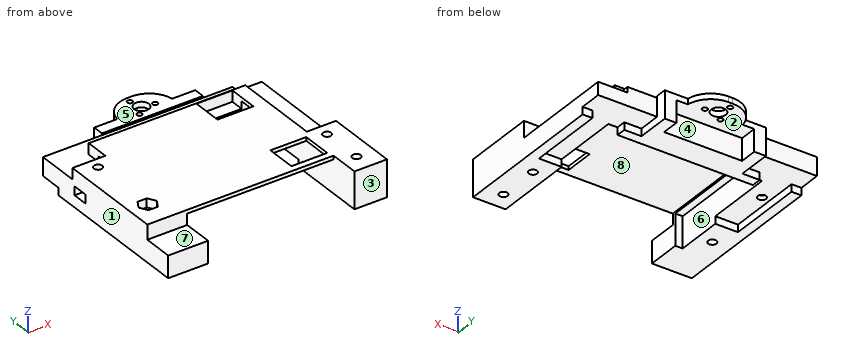
```python
from build123d import *

# Parameters (mm, degrees)
SKETCH1_R           = 6
BOSS_EXTRUDE1_DEPTH = 6
SKETCH2_W           = 27.6
SKETCH2_H           = 16.6
SKETCH2_R           = 6
SKETCH2_R_2         = 0.705
SKETCH2_R_3         = 2
BOSS_EXTRUDE2_DEPTH = 1.5
BOSS_EXTRUDE3_START = -4
BOSS_EXTRUDE3_DEPTH = 4
SKETCH5_W           = 40
SKETCH5_H           = 38.75
CUT_EXTRUDE1_DEPTH  = 50.346876803
SKETCH6_W           = 59.8
SKETCH6_H           = 40.75
BOSS_EXTRUDE4_DEPTH = 4
SKETCH7_W           = 40
SKETCH7_H           = 38.75
CUT_EXTRUDE2_DEPTH  = 3
SKETCH8_W           = 10.5
SKETCH8_H           = 8.15
CUT_EXTRUDE3_DEPTH  = 3
SKETCH8_3_W         = 9.813424901
SKETCH8_3_H         = 8.2
CUT_EXTRUDE4_DEPTH  = 1
CUT_EXTRUDE5_DEPTH  = 2
SKETCH10_W          = 8.9
SKETCH10_H          = 8.15
BOSS_EXTRUDE5_DEPTH = 4
SKETCH12_W          = 7.5
SKETCH12_H          = 1.5
CUT_EXTRUDE7_DEPTH  = 50.346876803
CUT_EXTRUDE8_DEPTH  = 2.4
CUT_EXTRUDE9_DEPTH  = 2.4
SKETCH16_R          = 1.125
CUT_EXTRUDE10_DEPTH = 50.788193884
SKETCH17_W          = 42
SKETCH17_H          = 31
CUT_EXTRUDE11_DEPTH = 8.5
SKETCH19_W          = 21.3
SKETCH19_H          = 12.25
CUT_EXTRUDE12_DEPTH = 50.141268301
SKETCH20_W          = 3.149886021
SKETCH20_H          = 7.5
SKETCH20_W_2        = 3.150113979
CUT_EXTRUDE13_DEPTH = 50.346876803
FILLET1_R           = 7
SKETCH21_W          = 5
SKETCH21_H          = 1.4
CUT_EXTRUDE14_DEPTH = 50.141268301
SKETCH22_W          = 9.813424901
SKETCH22_H          = 3.6
CUT_EXTRUDE15_DEPTH = 2
SKETCH23_W          = 3.149886021
SKETCH23_H          = 7.5
SKETCH23_W_2        = 3.150113979
CUT_EXTRUDE16_DEPTH = 50.346876803
SKETCH24_W          = 35
SKETCH24_H          = 1.4
CUT_EXTRUDE17_DEPTH = 49.713519689


# Read off the part's stored shape, not the designer's step: Boss-Extrude3
with BuildPart() as part:
    # Sketch1 → Boss-Extrude1 (new body)
    with BuildSketch(Plane.XY):
        Polygon((-10.832250172, 36.035749909), (-10.832250172, 19.435749909), (-15.532250172, 19.435749909), (-15.532250172, -1.464250091), (-24.232250172, -1.464250091), (-24.232250172, 19.435749909), (-26.932250172, 19.435749909), (-26.932250172, -23.364250091), (32.867749828, -23.364250091), (32.867749828, 19.435749909), (30.167749828, 19.435749909), (30.167749828, -1.464250091), (21.467749828, -1.464250091), (21.467749828, 19.435749909), (16.767749828, 19.435749909), (16.767749828, 36.035749909), align=None)
        with Locations((2.967749828, 29.785749909)):
            Circle(SKETCH1_R, mode=Mode.SUBTRACT)
    extrude(amount=BOSS_EXTRUDE1_DEPTH)

    # Sketch2 → Boss-Extrude2 (add)
    # profile 1 of 2: a face of its own
    with BuildSketch(Plane.XY.offset(6)):
        with Locations((2.967749828, 27.735749909)):
            Rectangle(SKETCH2_W, SKETCH2_H)
        with Locations((2.967749828, 29.785749909)):
            Circle(SKETCH2_R, mode=Mode.SUBTRACT)
    # profile 2 of 2: a face of its own
    with BuildSketch(Plane.XY.offset(6)):
        with Locations((2.967749828, 29.785749909)):
            Circle(SKETCH2_R)
        with Locations((0.732850657, 27.357741339)):
            Circle(SKETCH2_R_2, mode=Mode.SUBTRACT)
        with Locations((6.187916827, 29.064275155)):
            Circle(SKETCH2_R_2, mode=Mode.SUBTRACT)
        with Locations((1.982482071, 32.935233827)):
            Circle(SKETCH2_R_2, mode=Mode.SUBTRACT)
        with Locations((2.967749828, 29.785749909)):
            Circle(SKETCH2_R_3, mode=Mode.SUBTRACT)
    extrude(amount=BOSS_EXTRUDE2_DEPTH)

    # Boss-Extrude3 outline → Boss-Extrude3 (add)
    with BuildSketch(Plane.XY.offset(6).offset(BOSS_EXTRUDE3_START)):
        Polygon((32.867749828, 19.435749909), (32.867749828, 25.535749909), (16.767749828, 25.535749909), (16.767749828, 19.435749909), (21.467749828, 19.435749909), (21.467749828, -1.464250091), (30.167749828, -1.464250091), (30.167749828, 19.435749909), align=None)
        Polygon((-26.932250172, 25.535749909), (-26.932250172, 19.435749909), (-24.232250172, 19.435749909), (-24.232250172, -1.464250091), (-15.532250172, -1.464250091), (-15.532250172, 19.435749909), (-10.832250172, 19.435749909), (-10.832250172, 25.535749909), align=None)
    extrude(amount=BOSS_EXTRUDE3_DEPTH)

    # Sketch5 → Cut-Extrude1 (cut, through all)
    with BuildSketch(Plane(origin=(0, 0, 0), x_dir=(-1, 0, 0), z_dir=(0, 0, -1))):
        with Locations((-3.967749828, -2.589250091)):
            Rectangle(SKETCH5_W, SKETCH5_H)
    extrude(amount=-CUT_EXTRUDE1_DEPTH, mode=Mode.SUBTRACT)

    # Sketch6 → Boss-Extrude4 (add)
    with BuildSketch(Plane.XY.offset(6)):
        with Locations((2.967749828, 5.160749909)):
            Rectangle(SKETCH6_W, SKETCH6_H)
    extrude(amount=BOSS_EXTRUDE4_DEPTH)

    # Sketch7 → Cut-Extrude2 (cut)
    with BuildSketch(Plane(origin=(0, 0, 6), x_dir=(-1, 0, 0), z_dir=(0, 0, -1))):
        with Locations((-3.967749828, -2.589250091)):
            Rectangle(SKETCH7_W, SKETCH7_H)
    extrude(amount=-CUT_EXTRUDE2_DEPTH, mode=Mode.SUBTRACT)

    # Sketch8 → Cut-Extrude3 (cut)
    with BuildSketch(Plane.XY.offset(10)):
        Polygon((24.867749828, -3.464250091), (32.867749828, -3.464250091), (32.867749828, 25.535749909), (-26.932250172, 25.535749909), (-26.932250172, 14.035749909), (-17.932250172, 14.035749909), (-17.932250172, 20.535749909), (24.867749828, 20.535749909), align=None)
        with Locations((-21.682250172, -19.289250091)):
            Rectangle(SKETCH8_W, SKETCH8_H)
    extrude(amount=-CUT_EXTRUDE3_DEPTH, mode=Mode.SUBTRACT)

    # Sketch8<3> → Cut-Extrude4 (cut)
    with BuildSketch(Plane.XY.offset(10)):
        with Locations((16.317749828, 16.285749909)):
            Rectangle(SKETCH8_3_W, SKETCH8_3_H)
        with Locations((18.567749828, -9.364250091)):
            Rectangle(SKETCH8_3_W, SKETCH8_3_H)
    extrude(amount=-CUT_EXTRUDE4_DEPTH, mode=Mode.SUBTRACT)

    # Sketch9 → Cut-Extrude5 (cut)
    with BuildSketch(Plane.XY.offset(7.5)):
        Polygon((24.867749828, 20.535749909), (24.867749828, -3.464250091), (32.867749828, -3.464250091), (32.867749828, 25.535749909), (24.867749828, 25.535749909), align=None)
    extrude(amount=-CUT_EXTRUDE5_DEPTH, mode=Mode.SUBTRACT)

    # Sketch10 → Boss-Extrude5 (add)
    with BuildSketch(Plane.XY.offset(6)):
        with Locations((28.417749828, -19.289250091)):
            Rectangle(SKETCH10_W, SKETCH10_H)
    extrude(amount=BOSS_EXTRUDE5_DEPTH)

    # Sketch12 → Cut-Extrude7 (cut, through all)
    with BuildSketch(Plane.XY.offset(7.5)):
        with Locations((-0.78247813, 35.285749909)):
            Rectangle(SKETCH12_W, SKETCH12_H)
        with Locations((6.71752187, 35.285749909)):
            Rectangle(SKETCH12_W, SKETCH12_H)
    extrude(amount=-CUT_EXTRUDE7_DEPTH, mode=Mode.SUBTRACT)

    # Sketch13 → Cut-Extrude8 (cut)
    with BuildSketch(Plane.XY.offset(10)):
        Polygon((-19.432250172, -8.214250091), (-20.682250172, -6.049186582), (-23.182250172, -6.049186582), (-24.432250172, -8.214250091), (-23.182250172, -10.379313601), (-20.682250172, -10.379313601), align=None)
    extrude(amount=-CUT_EXTRUDE8_DEPTH, mode=Mode.SUBTRACT)

    # Sketch15 → Cut-Extrude9 (cut)
    with BuildSketch(Plane(origin=(-203.37180159, 125.682543488, 5.600198), x_dir=(1, 0, 0), z_dir=(0, 0, 1))):
        Polygon((180.089551417, -116.811857089), (182.589551417, -116.811857089), (183.839551417, -114.646793579), (182.589551417, -112.48173007), (180.089551417, -112.48173007), (178.839551417, -114.646793579), align=None)
        Polygon((176.439551417, -112.48173007), (176.439551417, -116.811857089), (180.089551417, -116.811857089), (178.839551417, -114.646793579), (180.089551417, -112.48173007), align=None)
    extrude(amount=-CUT_EXTRUDE9_DEPTH, mode=Mode.SUBTRACT)

    # Sketch16 → Cut-Extrude10 (cut, through all)
    with BuildSketch(Plane.XY.offset(10)):
        with Locations((-21.932250172, -8.214250091)):
            Circle(SKETCH16_R)
        with Locations((-22.032250172, 11.035749909)):
            Circle(SKETCH16_R)
        with Locations((27.967749828, -6.964250091)):
            Circle(SKETCH16_R)
        with Locations((27.967749828, -18.464250091)):
            Circle(SKETCH16_R)
    extrude(amount=-CUT_EXTRUDE10_DEPTH, mode=Mode.SUBTRACT)

    # Sketch17 → Cut-Extrude11 (cut)
    with BuildSketch(Plane(origin=(0, 0, 0), x_dir=(-1, 0, 0), z_dir=(0, 0, -1))):
        with Locations((-2.967749828, 1.285749909)):
            Rectangle(SKETCH17_W, SKETCH17_H)
    extrude(amount=-CUT_EXTRUDE11_DEPTH, mode=Mode.SUBTRACT)

    # Sketch19 → Cut-Extrude12 (cut, through all)
    with BuildSketch(Plane(origin=(0, 0, 6), x_dir=(-1, 0, 0), z_dir=(0, 0, -1))):
        with Locations((-2.967635849, 29.910749909)):
            Rectangle(SKETCH19_W, SKETCH19_H)
    extrude(amount=CUT_EXTRUDE12_DEPTH, mode=Mode.SUBTRACT)

    # Sketch20 → Cut-Extrude13 (cut, through all)
    with BuildSketch(Plane.XY.offset(7.5)):
        with Locations((-6.107421141, 32.285749909)):
            Rectangle(SKETCH20_W, SKETCH20_H)
        with Locations((12.04257886, 32.285749909)):
            Rectangle(SKETCH20_W_2, SKETCH20_H)
    extrude(amount=-CUT_EXTRUDE13_DEPTH, mode=Mode.SUBTRACT)

    # Fillet1
    # the kernel refuses this fillet: 7 mm, written as the material it takes off along each edge
    with BuildSketch(Plane(origin=(-4.53247813, 34.535749909, 24.820508076), x_dir=(0, -1, 0), z_dir=(0, 0, -1))) as fillet1_piece_1:
        with BuildLine():
            CenterArc((7, -6.92820323), FILLET1_R, 98.213210702, 81.786789298)
            Line((0, -6.92820323), (-0.14, -6.92820323))
            Line((-0.14, -6.92820323), (-0.14, 0))
            Line((-0.14, 0), (0, 0.14))
            ThreePointArc((0, 0.14), (3, 0.14), (5.98, 0.138564065))
            Line((5.98, 0.138564065), (6, 0))
        make_face()
    extrude(amount=36.141016151, mode=Mode.SUBTRACT)
    with BuildSketch(Plane(origin=(10.46752187, 34.535749909, 24.820508076), x_dir=(-1, 0, 0), z_dir=(0, 0, -1))) as fillet1_piece_2:
        with BuildLine():
            CenterArc((6.92820323, -7), FILLET1_R, 90, 81.786789298)
            Line((0, -6), (-0.138564065, -5.98))
            ThreePointArc((-0.138564065, -5.98), (-0.14, -3), (-0.14, 0))
            Line((-0.14, 0), (0, 0.14))
            Line((0, 0.14), (6.92820323, 0.14))
            Line((6.92820323, 0.14), (6.92820323, 0))
        make_face()
    extrude(amount=36.141016151, mode=Mode.SUBTRACT)

    # Sketch21 → Cut-Extrude14 (cut, through all)
    with BuildSketch(Plane.XY.offset(6)):
        with Locations((-13.532250172, -22.664250091)):
            Rectangle(SKETCH21_W, SKETCH21_H)
    extrude(amount=-CUT_EXTRUDE14_DEPTH, mode=Mode.SUBTRACT)

    # Sketch22 → Cut-Extrude15 (cut)
    with BuildSketch(Plane.XY.offset(9)):
        with Locations((16.317749828, 18.585749909)):
            Rectangle(SKETCH22_W, SKETCH22_H)
    extrude(amount=-CUT_EXTRUDE15_DEPTH, mode=Mode.SUBTRACT)

    # Sketch23 → Cut-Extrude16 (cut, through all)
    with BuildSketch(Plane.XY.offset(7.5)):
        with Locations((-9.257307161, 32.285749909)):
            Rectangle(SKETCH23_W, SKETCH23_H)
        with Locations((15.192692839, 32.285749909)):
            Rectangle(SKETCH23_W_2, SKETCH23_H)
    extrude(amount=-CUT_EXTRUDE16_DEPTH, mode=Mode.SUBTRACT)

    # Sketch24 → Cut-Extrude17 (cut, through all)
    with BuildSketch(Plane(origin=(0, 0, 0), x_dir=(-1, 0, 0), z_dir=(0, 0, -1))):
        with Locations((-6.467749828, -22.664250091)):
            Rectangle(SKETCH24_W, SKETCH24_H)
    extrude(amount=-CUT_EXTRUDE17_DEPTH, mode=Mode.SUBTRACT)


solid = part.part
```
Could you check a few things on this model? Use its own coordinates, in mm. Face numbers are marked on the shaded views. A direction names the side the tool comes from. Round coordinates to 2 decimals unless told otherwise and drop trailing zeros. Loops run counter-clockwise (first coordinate to the right, second up) from the corner with the lowest first, then second, coordinate; pieces in that order, holes last. Notation, with made-up numbers: (85, 38.25) -> (102, 38.25) arc R31 ccw to (102, 68.25) -> close; hole circle Ø7 at (-14, 37.25). An arc over 180 degrees is marked (long way). Put each result on its own line as item: value.
Q1. Please list where these lines run through material, in increasing order: line 1 (X direction, y = 18, z = 1.5); line 2 (X direction, y = 24.5, z = 2.25); line 3 (X direction, y = 8.5, z = 1.25). Write a range as from..to.
Checks:
line 1: -26.93..-24.23, -15.53..21.47, 30.17..32.87
line 2: -26.93..-7.68, 13.62..32.87
line 3: -26.93..-24.23, 30.17..32.87
Q2. For pin 1 Ø1.5 at (x, z) = (-2, 8) entering from +Y; pin 2 Ø1.1 at (x, y) = (17, 19.5) entering from +Z; pin 3 Ø2 at (x, z) = (5, 6.5) entering from -Y, each with a flat end and sliding along its axis, tell me the tip position at first contact or that it passes through.
Checks:
pin 1: y = 33.39
pin 2: z = 7
pin 3: y = 16.79
Q3. I want a section at C-C on y = 2.5. Write out the boundary of the cut face in (x, z), and give its area (3 significant figures).
Checks:
outline: (-26.93, 0) -> (-24.23, 0) -> (-24.23, 2) -> (-18.03, 2) -> (-18.03, 8.5) -> (-16.03, 8.5) -> (-16.03, 9) -> (23.97, 9) -> (23.97, 2) -> (30.17, 2) -> (30.17, 0) -> (32.87, 0) -> (32.87, 5.5) -> (24.87, 5.5) -> (24.87, 10) -> (-26.93, 10) -> close
area: 160 mm2
Q4. I want a section at D-D on x = 12.5. Write out the boundary of the cut face in (y, z), and give its area (3 significant figures).
Checks:
outline: (-15.21, 9) -> (12.19, 9) -> (12.19, 10) -> (-15.21, 10) -> close; (16.79, 0) -> (23.79, 0) -> (23.79, 6) -> (28.54, 6) -> (28.54, 7.5) -> (25.54, 7.5) -> (25.54, 7) -> (20.54, 7) -> (20.54, 10) -> (20.39, 10) -> (20.39, 7) -> (16.79, 7) -> close
area: 83.1 mm2
Q5. Which directions (+Z, -Z, +X, -X, +Y, -Y) give clear straight access to the entire face, cutting with the end or side of a thin tool? Please do the marked faces 4, 5, 6, 7 and 8.
Checks:
face 4: -Z, +Y
face 5: +Z, +X, -X, +Y
face 6: -Z
face 7: +Z, -X, -Y
face 8: -Z, -Y
Q6. Thinking about a two-plate mould opening in X: for the marked faces 1, 2 and 3, which applies, pulls with the +X half, pulls with the -X half, needs draft (parallel to the pull), parting line crosses it, or undercut?
Checks:
face 1: pulls with the -X half
face 2: undercut
face 3: needs draft
Q7. I want a section at B-B on x = 18.5. Write out the boundary of the cut face in (y, z), and give its area (3 significant figures).
Checks:
outline: (-15.21, 9) -> (-13.46, 9) -> (-13.46, 10) -> (-15.21, 10) -> close; (-5.26, 9) -> (12.19, 9) -> (12.19, 10) -> (-5.26, 10) -> close; (16.79, 0) -> (19.44, 0) -> (19.44, 2) -> (25.54, 2) -> (25.54, 7) -> (20.54, 7) -> (20.54, 10) -> (20.39, 10) -> (20.39, 7) -> (16.79, 7) -> close
area: 68.7 mm2
Q8. I want a section at A-A on z = 1.25. Give the number of separate pieces and of enclosed holes in the cut face, and give its area (3 significant figures).
Checks:
separate pieces: 3
enclosed holes: 3
area: 757 mm2
